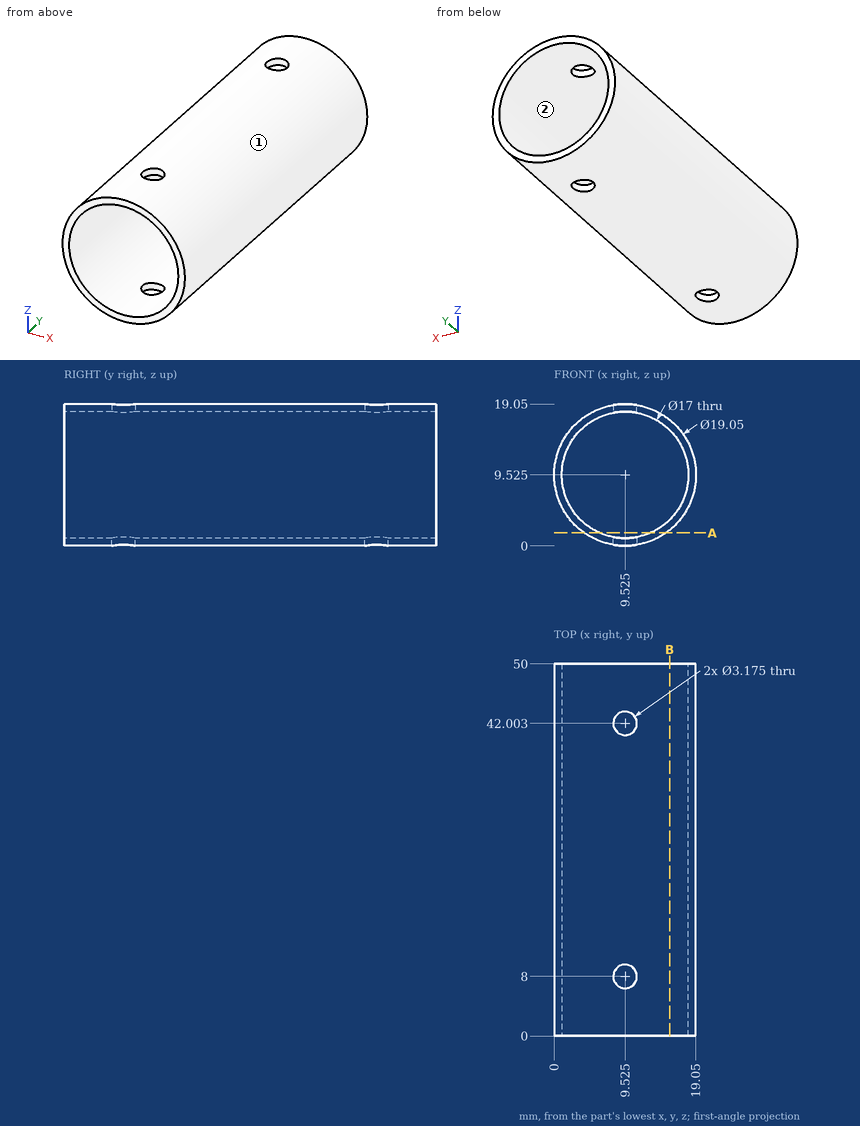
The drawing under review shows one solid part. Ordinate dimensions are in mm from its lowest x, y, z. Give positions to 0.01 mm unless a question says otherwise; leave off trailing zeros. Write each loop counter-clockwise with the first axis right and the second up, starting at its lowest first coordinate (ties: lowest second). Pieces come first, ordered by that corner, then holes. Notation, with made-up numbers: (-10.5, 72) -> (20.5, 72) arc R25 ccw to (20.5, 99) -> close; hole circle Ø2 at (36.5, 36.5). An arc over 180 degrees is marked (long way). Use CSV: the item, a comma, the result in double quotes.
Q1. Take a section at B-B, the plane x = 15.5. Write out the cut boundary in (y, z).
Conclusion:
outline,"(0, 2.11) -> (50, 2.11) -> (50, 3.48) -> (0, 3.48) -> close; (0, 15.57) -> (50, 15.57) -> (50, 16.94) -> (0, 16.94) -> close"
Q2. Take a section at A-A, the plane z = 1.75. Write out the cut boundary in (x, y), then the cut area to 3 significant figures.
Conclusion:
outline,"(4.02, 0) -> (6.09, 0) -> (6.09, 50) -> (4.02, 50) -> close; (12.96, 0) -> (15.03, 0) -> (15.03, 50) -> (12.96, 50) -> close"
area,"207 mm2"
Q3. For P1, Ø4, axis at x = 14, y = 29.5, coming from the -Z side; P2, Ø1, axis at y = 19.5, z = 13, coming from the +X side; P3, Ø1.5, axis at y = 44, z = 11.5, coming from the -X side, all flat-tipped, find the tip position at first contact; note any pin that passes through.
Conclusion:
P1,"z = 0.33"
P2,"x = 18.57"
P3,"x = 0.08"
Q4. Mouldability with a two-part tool opening along X and no side actions: class the marked faces 1 and 2 as pulls with the +X half, pulls with the -X half, needs draft (parallel to the pull), parting line crosses it, or undercut.
Conclusion:
face 1,"parting line crosses it"
face 2,"undercut"
Q5. To check wall thickness, follow probe 1 along X at (y, z) = (30.5, 9.25) (1 decimal); probe 2 along Z at (x, y) = (10.25, 12.5) (1 decimal); probe 3 along X at (y, z) = (9.5, 17) (1 decimal). State the ranges of each line that lie inside material, in increasing order. Write a range as [from, to].
Conclusion:
probe 1,"[0, 1], [18, 19]"
probe 2,"[0, 1.1], [18, 19]"
probe 3,"[3.6, 5.5], [13.6, 15.4]"
